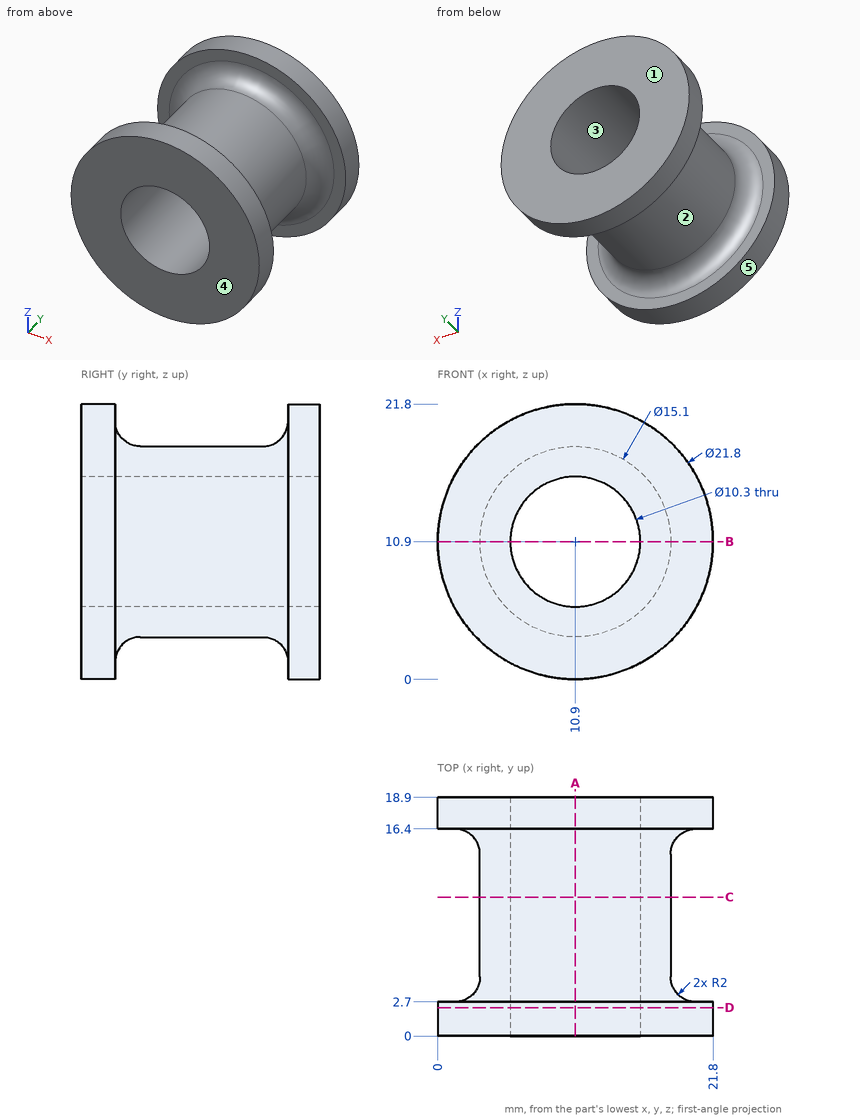
For this review, use the dimensioned drawing (mm, ordinates from the lowest corner) and the shaded views. A direction names the side the tool comes from. Coordinates: 2 decimals unless noted, no trailing zeros. Write each loop counter-clockwise with the first axis right and the second up, starting at its lowest first coordinate (ties: lowest second). Pieces come first, ordered by that corner, then holes. Notation, with made-up numbers: (87, -17) - (124, -17) arc R17 ccw to (124, -7) - close; hole circle Ø4 at (76.5, 44.5). An arc over 180 degrees is marked (long way). Answer in a Markdown table with one row per item. Add a question column.
Q1. Consider section B-B on z = 10.9. Give the boundary of the cut face in (x, y).
Q2. For the marked faces 1 and 2, list the 3-axis set-ups (+Z, -Z, +X, -X, +Y, -Y) from which the entire face can be reached by the end or side of a thin tool; tool diameter is ignored.
Q3. Consider section D-D on y = 2.25. Give the boundary of the cut face in (x, z), then the cut area to 3 significant figures.
Q4. Draft analysis for pull direction Z (two halves, no side actions). For the marked faces 3, 4 and 5, state which applies: +Z half, -Z half, draft (parallel to the pull), parting line (faces both ways), or undercut.
Q5. Consider section A-A on x = 10.9. Give the boundary of the cut face in (y, z).
Q6. To check wall thickness, follow line 1 along Y through (x, z) = (7, 20.75); line 2 along Z through (x, y) = (10.9, 12.75); line 3 along Z through (x, y) = (11, 1.25). State the ranges of each line that lie inside material, in increasing order. Write a range as from..to.
Q7. Clearance check with flat-ended pins moving along their axes: pin 1 (4 mm diameter, centred on x = 6.5, y = 11.5, fed in from -Z); pin 2 (1.5 mm diameter, centred on y = 7, z = 8.5, fed in from +X); pin 3 (5 mm diameter, centred on y = 13, z = 19.5, fed in from +X). State where each tip first meets the part, or that it passes through.
Q8. Consider section C-C on y = 11. Give the boundary of the cut face in (x, z), then the cut area to 3 significant figures.
Answers below:
| question | item | result |
|---|---|---|
| 1 | outline | (0, 0) - (5.75, 0) - (5.75, 18.9) - (0, 18.9) - (0, 16.4) - (1.35, 16.4) arc R2 cw to (3.35, 14.4) - (3.35, 4.7) arc R2 cw to (1.35, 2.7) - (0, 2.7) - close; (16.05, 0) - (21.8, 0) - (21.8, 2.7) - (20.45, 2.7) arc R2 cw to (18.45, 4.7) - (18.45, 14.4) arc R2 cw to (20.45, 16.4) - (21.8, 16.4) - (21.8, 18.9) - (16.05, 18.9) - close |
| 2 | face 1 | +Z, -Z, +X, -X, +Y |
| 2 | face 2 | none |
| 3 | outline | circle Ø21.8 at (10.9, 10.9); hole circle Ø10.3 at (10.9, 10.9) |
| 3 | area | 290 mm² |
| 4 | face 3 | undercut |
| 4 | face 4 | draft |
| 4 | face 5 | parting line |
| 5 | outline | (0, 0) - (2.7, 0) - (2.7, 1.35) arc R2 cw to (4.7, 3.35) - (14.4, 3.35) arc R2 cw to (16.4, 1.35) - (16.4, 0) - (18.9, 0) - (18.9, 5.75) - (0, 5.75) - close; (0, 16.05) - (18.9, 16.05) - (18.9, 21.8) - (16.4, 21.8) - (16.4, 20.45) arc R2 cw to (14.4, 18.45) - (4.7, 18.45) arc R2 cw to (2.7, 20.45) - (2.7, 21.8) - (0, 21.8) - close |
| 6 | line 1 | 0..2.7, 16.4..18.9 |
| 6 | line 2 | 3.35..5.75, 16.05..18.45 |
| 6 | line 3 | 0..5.75, 16.05..21.8 |
| 7 | pin 1 | z = 3.74 |
| 7 | pin 2 | x = 18.27 |
| 7 | pin 3 | x = 15.35 |
| 8 | outline | circle Ø15.1 at (10.9, 10.9); hole circle Ø10.3 at (10.9, 10.9) |
| 8 | area | 95.8 mm² |
